```python
from build123d import *

# Parameters (mm, degrees)
F0_R     = 87.5
F1_DEPTH = 2


# Not quite as in the source:
# - a feature of the source that left no trace in its solid (it failed there, or was rolled back) is left out


with BuildPart() as f1:
    # F0 (on Front) → F1 (new body)
    with BuildSketch(Plane.XZ):
        Circle(F0_R)
        with BuildLine():
            ThreePointArc((-53.8334623112, -64.1562221112), (-59.2201929244, -59.2201929244), (-64.1562221112, -53.8334623112))
            Line((-64.1562221112, -53.8334623112), (-62.2411110034, -52.226493287))
            ThreePointArc((-62.2411110034, -52.226493287), (-57.4524259714, -57.4524259714), (-52.226493287, -62.2411110034))
            Line((-52.226493287, -62.2411110034), (-53.8334623112, -64.1562221112))
        make_face(mode=Mode.SUBTRACT)
        with BuildLine():
            Line((53.8334623112, -64.1562221112), (52.226493287, -62.2411110034))
            ThreePointArc((52.226493287, -62.2411110034), (57.4524259714, -57.4524259714), (62.2411110034, -52.226493287))
            Line((62.2411110034, -52.226493287), (64.1562221112, -53.8334623112))
            ThreePointArc((64.1562221112, -53.8334623112), (59.2201929244, -59.2201929244), (53.8334623112, -64.1562221112))
        make_face(mode=Mode.SUBTRACT)
        Polygon((-45, 15), (-45, 0), (-45, -15), (-51, -15), (-51, 15), align=None, mode=Mode.SUBTRACT)
        with BuildLine():
            ThreePointArc((-64.1562221112, 53.8334623112), (-59.2201929244, 59.2201929244), (-53.8334623112, 64.1562221112))
            Line((-53.8334623112, 64.1562221112), (-52.226493287, 62.2411110034))
            ThreePointArc((-52.226493287, 62.2411110034), (-57.4524259714, 57.4524259714), (-62.2411110034, 52.226493287))
            Line((-62.2411110034, 52.226493287), (-64.1562221112, 53.8334623112))
        make_face(mode=Mode.SUBTRACT)
        Polygon((51, 15), (51, -15), (45, -15), (45, 0), (45, 15), align=None, mode=Mode.SUBTRACT)
        with BuildLine():
            ThreePointArc((53.8334623112, 64.1562221112), (59.2201929244, 59.2201929244), (64.1562221112, 53.8334623112))
            Line((64.1562221112, 53.8334623112), (62.2411110034, 52.226493287))
            ThreePointArc((62.2411110034, 52.226493287), (57.4524259714, 57.4524259714), (52.226493287, 62.2411110034))
            Line((52.226493287, 62.2411110034), (53.8334623112, 64.1562221112))
        make_face(mode=Mode.SUBTRACT)
    extrude(amount=-F1_DEPTH)


solid = f1.part
```
Check sheet for the modelled part. Datum: model origin and axes. Units: mm. A direction names the side the tool comes from. Give positions to 0.01 mm unless a question says otherwise; leave off trailing zeros. Order: outer loops, then holes, each group sorted by start corner. A loop starts at its lowest first (then second) coordinate and runs counter-clockwise, first axis right, second up. Notation, with made-up numbers: M -6,2 L 51,2 A11 ccw 51,22 Z; hole C -12,4.25 d10. An arc over 180 degrees is marked long. Answer in a Markdown table with one row per item. Add a question column.
Q1. Sectioned sample at C-C, the plane z = 24.5. Record the boundary of the cut face in (x, y).
Q2. Release check for a two-part mould opening along Z. For faces 1 (the flat face through (-1, 2, 1)), 2 (the cylindrical face through (-59.15, 0.99, -59.29)), 3 (the cylindrical face through (-64.49, 0.99, 59.14)) record: released by +Z, released by -Z, zero draft, split by the parting line, or undercut.
Q3. Sectioned sample at A-A, the plane z = 0. Record the boundary of the cut face in (x, y), and give its area (3 significant figures).
Q4. Sectioned sample at D-D, the plane x = 21.5. Record the boundary of the cut face in (y, z).
Q5. Access from +Z, -Z, +X, -X, +Y, -Y to the whole of each face (thin tool, end or side, straight path). Record for faces 4 (the flat face through (-1, 0, 1)), 5 (the cylindrical face through (-57.382, 0.986, 57.523)).
Q6. Thickness scan on L1, parallel to Z at x = -59.5, y = 0.55; L2, parallel to X at y = 1.85, z = -13.5; L3, parallel to Z at x = -56, y = 1.3. Record the ranges inside material, lowest first.
Q7. Gauge pin test, flat ends, axial feed: pin 1 Ø0.6 at (y, z) = (0.5, 2) entering from +X; pin 2 Ø1 at (y, z) = (1, 24) entering from +X; pin 3 Ø0.6 at (x, y) = (47, 0.5) entering from -Z; pin 4 Ø8 at (x, z) = (22.5, -30) entering from -Y. Record the tip position at first contact, or that the pin passes through.
Q8. Sectioned sample at B-B, the plane y = 0.5. Record the boundary of the cut face in (x, z), and give its area (3 significant figures).
Verdict:
| question | item | result |
|---|---|---|
| 1 | outline | M -84,0 L 84,0 L 84,2 L -84,2 Z |
| 2 | face 1 | zero draft |
| 2 | face 2 | undercut |
| 2 | face 3 | split by the parting line |
| 3 | outline | M -87.5,0 L -51,0 L -51,2 L -87.5,2 Z; M -45,0 L 45,0 L 45,2 L -45,2 Z; M 51,0 L 87.5,0 L 87.5,2 L 51,2 Z |
| 3 | area | 326 mm² |
| 4 | outline | M 0,-84.82 L 2,-84.82 L 2,84.82 L 0,84.82 Z |
| 5 | face 4 | +Z, -Z, +X, -X, -Y |
| 5 | face 5 | +Y, -Y |
| 6 | L1 | -64.16 to -58.94, -55.33 to 55.33, 58.94 to 64.16 |
| 6 | L2 | -86.45 to -51, -45 to 45, 51 to 86.45 |
| 6 | L3 | -67.23 to -62.27, -58.87 to 58.87, 62.27 to 67.23 |
| 7 | pin 1 | x = 87.48 |
| 7 | pin 2 | x = 84.29 |
| 7 | pin 3 | z = -74 |
| 7 | pin 4 | y = 0 |
| 8 | outline | C 0,0 d175; hole M -64.16,-53.83 A83.75 ccw -53.83,-64.16 L -52.23,-62.24 A81.25 cw -62.24,-52.23 Z; hole M -64.16,53.83 L -62.24,52.23 A81.25 cw -52.23,62.24 L -53.83,64.16 A83.75 ccw Z; hole M -51,-15 L -45,-15 L -45,15 L -51,15 Z; hole M 45,-15 L 51,-15 L 51,15 L 45,15 Z; hole M 52.23,-62.24 L 53.83,-64.16 A83.75 ccw 64.16,-53.83 L 62.24,-52.23 A81.25 cw Z; hole M 52.23,62.24 A81.25 cw 62.24,52.23 L 64.16,53.83 A83.75 ccw 53.83,64.16 Z |
| 8 | area | 23,500 mm² |
